Can you work these out from the model? Positions are in its coordinate system, mm. Face numbers are marked on the shaded views. A direction names the side the tool comes from. Coordinates: 2 decimals unless noted, no trailing zeros. Order: outer loops, then holes, each group sorted by start corner. A loop starts at its lowest first (then second) coordinate and runs counter-clockwise, first axis right, second up.
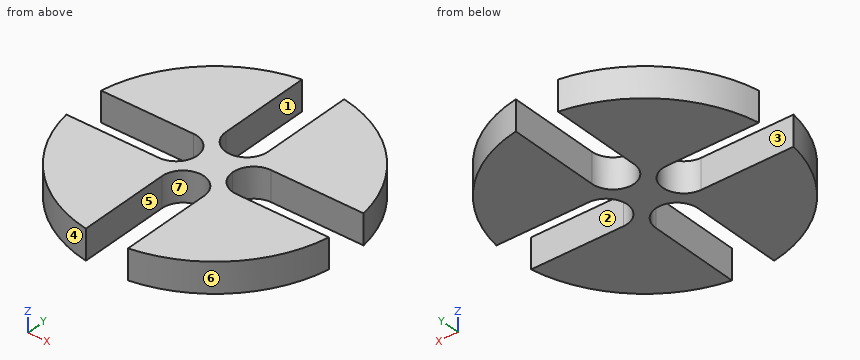
```python
from build123d import *

# Parameters (mm, degrees)
F1_DEPTH = 17


# Not quite as in the source:
# - a feature of the source that left no trace in its solid (it failed there, or was rolled back) is left out


with BuildPart() as f1:
    # F0 (on Top) → F1 (new body)
    with BuildSketch(Plane.XY):
        with BuildLine():
            Line((21.9, 11.9), (74.0499155975, 11.9))
            ThreePointArc((74.0499155975, 11.9), (53.033008589, 53.033008589), (11.9, 74.0499155975))
            Line((11.9, 74.0499155975), (11.9, 21.9))
            ThreePointArc((11.9, 21.9), (0, 10), (-11.9, 21.9))
            Line((-11.9, 21.9), (-11.9, 74.0499155975))
            ThreePointArc((-11.9, 74.0499155975), (-53.033008589, 53.033008589), (-74.0499155975, 11.9))
            Line((-74.0499155975, 11.9), (-21.9, 11.9))
            ThreePointArc((-21.9, 11.9), (-10, 0), (-21.9, -11.9))
            Line((-21.9, -11.9), (-74.0499155975, -11.9))
            ThreePointArc((-74.0499155975, -11.9), (-53.033008589, -53.033008589), (-11.9, -74.0499155975))
            Line((-11.9, -74.0499155975), (-11.9, -21.9))
            ThreePointArc((-11.9, -21.9), (0, -10), (11.9, -21.9))
            Line((11.9, -21.9), (11.9, -74.0499155975))
            ThreePointArc((11.9, -74.0499155975), (53.033008589, -53.033008589), (74.0499155975, -11.9))
            Line((74.0499155975, -11.9), (21.9, -11.9))
            ThreePointArc((21.9, -11.9), (13.4854293039, -8.4145706961), (10, 0))
            ThreePointArc((10, 0), (13.4854293039, 8.4145706961), (21.9, 11.9))
        make_face()
    extrude(amount=F1_DEPTH)


solid = f1.part
```
1. On a 3-axis mill with a long thin cutter (end or side, diameter ignored), from which of +Z, -Z, +X, -X, +Y, -Y can I reach the whole of each face in a straight line? I mean the marked faces 1, 2 and 3. Say none if no direction works.
Completed:
face 1: +Z, -Z, +Y
face 2: +Z, -Z, +X
face 3: +Z, -Z, -X
2. Imagine slicing it at B-B on y = 38.5. Please give me the cut outline in (x, z), then the cut area to 3 significant figures.
Completed:
outline: (-64.36, 0) - (-11.9, 0) - (-11.9, 17) - (-64.36, 17) - close; (11.9, 0) - (64.36, 0) - (64.36, 17) - (11.9, 17) - close
area: 1,780 mm2
3. Imagine slicing it at A-A on x = -59.5. Please give me the cut outline in (y, z).
Completed:
outline: (-45.66, 0) - (-11.9, 0) - (-11.9, 17) - (-45.66, 17) - close; (11.9, 0) - (45.66, 0) - (45.66, 17) - (11.9, 17) - close
4. Please list where these lines run through material, in increasing order: probe 1 along X at (y, z) = (0.5, 5); probe 2 along X at (y, z) = (-32.5, 14.25); probe 3 along X at (y, z) = (-13.5, 13.25) (3 decimals).
Completed:
probe 1: x = -10.01 to 10.01
probe 2: x = -67.59 to -11.9, 11.9 to 67.59
probe 3: x = -73.775 to -8.429, 8.429 to 73.775
5. I'm going to push flat-ended pins straight in: pin 1 (3 mm diameter, centred on y = -14.5, z = 15, fed in from -X); pin 2 (4 mm diameter, centred on x = -13, z = 14, fed in from -Y); pin 3 (4 mm diameter, centred on y = 27, z = 2, fed in from +X); pin 4 (4 mm diameter, centred on x = -51, z = 10.5, fed in from +Y). Where does each tip first touch, or does it pass through?
Completed:
pin 1: stops at x = -73.86
pin 2: stops at y = -74.05
pin 3: stops at x = 70.71
pin 4: stops at y = 56.78
6. Thinking about a two-plate mould opening in X: for the marked faces 4, 5, 6 and 7, which applies, pulls with the +X half, pulls with the -X half, needs draft (parallel to the pull), parting line crosses it, or undercut?
Completed:
face 4: pulls with the -X half
face 5: undercut
face 6: pulls with the +X half
face 7: undercut
7. Imagine slicing it at D-D on x = 0. Please give me the cut outline in (y, z).
Completed:
outline: (-10, 0) - (10, 0) - (10, 17) - (-10, 17) - close
8. Imagine slicing it at C-C on z = 8.25. Please give me the cut outline in (x, y), then the cut area to 3 significant figures.
Completed:
outline: (-74.05, -11.9) arc R75 ccw to (-11.9, -74.05) - (-11.9, -21.9) arc R11.9 cw to (11.9, -21.9) - (11.9, -74.05) arc R75 ccw to (74.05, -11.9) - (21.9, -11.9) arc R11.9 cw to (21.9, 11.9) - (74.05, 11.9) arc R75 ccw to (11.9, 74.05) - (11.9, 21.9) arc R11.9 cw to (-11.9, 21.9) - (-11.9, 74.05) arc R75 ccw to (-74.05, 11.9) - (-21.9, 11.9) arc R11.9 cw to (-21.9, -11.9) - close
area: 11,800 mm2
